from build123d import *

# Parameters (mm, degrees)
SKETCH1_R           = 0.635
BOSS_EXTRUDE1_DEPTH = 21.9456
SKETCH2_R           = 2.38125
SKETCH2_R_2         = 0.635
BOSS_EXTRUDE2_DEPTH = 4.9784
SKETCH3_R           = 2.38125
SKETCH3_R_2         = 0.635
BOSS_EXTRUDE3_DEPTH = 4.9784


with BuildPart() as part:
    # Sketch1 → Boss-Extrude1 (new body, symmetric)
    with BuildSketch(Plane(origin=(0, 0, 0), x_dir=(1, 0, 0), z_dir=(0, 1, 0))):
        Polygon((1.374815329, -2.38125), (2.749630657, 0), (1.374815329, 2.38125), (-1.374815329, 2.38125), (-2.749630657, 0), (-1.374815329, -2.38125), align=None)
        Circle(SKETCH1_R, mode=Mode.SUBTRACT)
    extrude(amount=BOSS_EXTRUDE1_DEPTH, both=True)

    # Sketch2 → Boss-Extrude2 (add)
    with BuildSketch(Plane(origin=(0, 21.9456, 0), x_dir=(1, 0, 0), z_dir=(0, 1, 0))):
        Circle(SKETCH2_R)
        Circle(SKETCH2_R_2, mode=Mode.SUBTRACT)
    extrude(amount=BOSS_EXTRUDE2_DEPTH)

    # Sketch3 → Boss-Extrude3 (add)
    with BuildSketch(Plane.XZ.offset(21.9456)):
        Circle(SKETCH3_R)
        Circle(SKETCH3_R_2, mode=Mode.SUBTRACT)
    extrude(amount=BOSS_EXTRUDE3_DEPTH)


solid = part.part
Read the model definition and answer for the solid it produces. Units are mm, in the model's axes. A direction names the side the tool comes from. Round coordinates to 2 decimals unless told otherwise and drop trailing zeros. Write each loop counter-clockwise with the first axis right and the second up, starting at its lowest first coordinate (ties: lowest second). Pieces come first, ordered by that corner, then holes.
1. Determine the mould class of faces 5 (the face through (-1.3, 21.946, 2.2)), 6 (the face through (-0.08, 0.38, 0.63)), 7 (the face through (0, 0, 2.381)) for opening direction Z: pulls with the +Z half, pulls with the -Z half, needs draft (parallel to the pull), parting line crosses it, or undercut.
2. The part is cut by section A-A, the plane y = -3. Determine the outline of the cut face in (x, z) (3 decimals), then the cut area to 3 significant figures.
3. Given pin 1 Ø1 at (x, z) = (0, 0) entering from +Y; pin 2 Ø0.6 at (x, z) = (1.5, 2) entering from -Y; pin 3 Ø2 at (y, z) = (-18, 0.5) entering from +X, each flat-ended and moving along its own axis, determine where each tip first touches the part or whether it passes through.
4. Which of the six approach directions +Z, -Z, +X, -X, +Y, -Y give full straight-line access (tool end or side, diameter ignored) to faces 1 (the face through (-1.3, 21.946, -2.2)), 2 (the face through (1.3, -21.946, 2.2)), 3 (the face through (1.3, 21.946, -2.2)), 4 (the face through (-1.89, 24.4, 1.45))?
5. Straight lines are drawn through the part: L1, parallel to X at y = -11, z = 0 (3 decimals); L2, parallel to Z at x = 0, y = 7 (3 decimals); L3, parallel to X at y = 22, z = 0.05. For each, find the intervals that lie inside material, in ascending order.
6. The part is cut by section B-B, the plane z = 1.7. Determine the outline of the cut face in (x, y), then the cut area to 3 significant figures.
Values:
1. face 5: needs draft
1. face 6: undercut
1. face 7: pulls with the +Z half
2. outline: (-2.75, 0) - (-1.375, -2.381) - (1.375, -2.381) - (2.75, 0) - (1.375, 2.381) - (-1.375, 2.381) - close; hole circle Ø1.27 at (0, 0)
2. area: 18.4 mm2
3. pin 1: passes through
3. pin 2: stops at y = -26.92
3. pin 3: stops at x = 2.75
4. face 1: -Z, -X, +Y
4. face 2: +Z, +X, -Y
4. face 3: -Z, +X, +Y
4. face 4: +Y
5. L1: x = -2.75 to -0.635, 0.635 to 2.75
5. L2: z = -2.381 to -0.635, 0.635 to 2.381
5. L3: x = -2.38 to -0.63, 0.63 to 2.38
6. outline: (-1.77, -21.95) - (-1.67, -21.95) - (-1.67, -26.92) - (1.67, -26.92) - (1.67, -21.95) - (1.77, -21.95) - (1.77, 21.95) - (1.67, 21.95) - (1.67, 26.92) - (-1.67, 26.92) - (-1.67, 21.95) - (-1.77, 21.95) - close
6. area: 188 mm2
